For this review, use the dimensioned drawing (mm, ordinates from the lowest corner) and the shaded views. Round coordinates to 2 decimals unless told otherwise and drop trailing zeros. Loops run counter-clockwise (first coordinate to the right, second up) from the corner with the lowest first, then second, coordinate; pieces in that order, holes last. Notation, with made-up numbers: M 89,44 L 108,44 A29 cw 108,65 Z; hole C 72,31.25 d11. An arc over 180 degrees is marked long. Answer as a JSON object with one key per item and string values. Group by question number.
Item 1: Consider section B-B (x = 45). Give the boundary of the cut face in (y, z), and give its area (3 significant figures).
Item 2: Insertion check: P1, Ø1.2, axis at x = 60, y = 34, coming from the +Z side; P2, Ø2.5, axis at x = 115, y = 2, coming from the +Z side; P3, Ø0.8, axis at x = 68.5, z = 2.5, coming from the +Y side. Each pin has a flat end and moves straight along its axis. Give the tip position at first contact, or say it passes through.
Item 3: To check wall thickness, follow line 1 (X direction, y = 34, z = 0.8); line 2 (Y direction, x = 60, z = 1.6); line 3 (Z direction, x = 42, y = 4). State the ranges of each line that lie inside material, in increasing order.
Item 4: Consider section A-A (y = 8). Give the boundary of the cut face in (x, z).
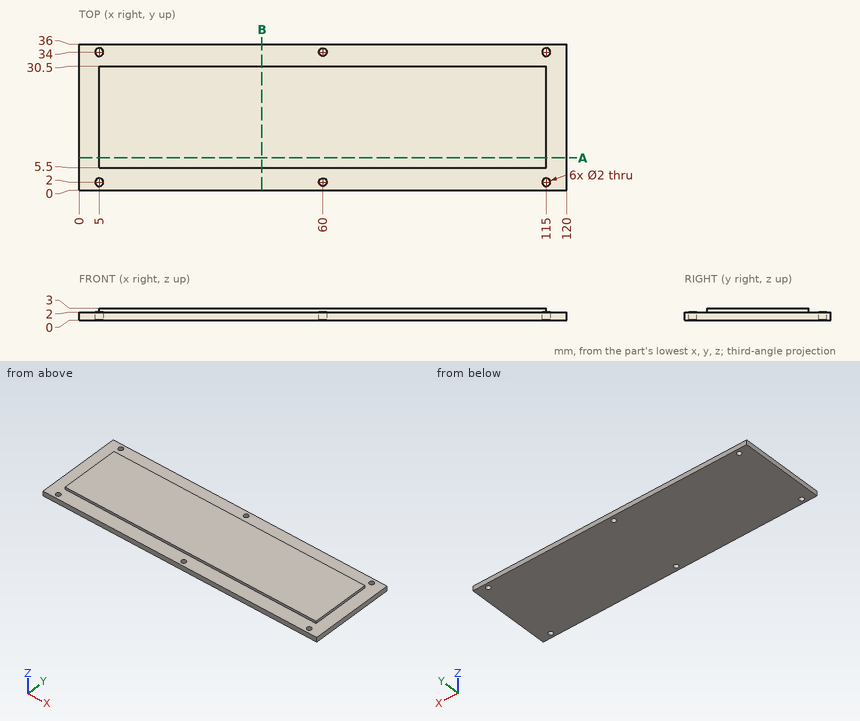
Geometry results:
{
 "1": {"outline": "M 0,0 L 36,0 L 36,2 L 30.5,2 L 30.5,3 L 5.5,3 L 5.5,2 L 0,2 Z", "area": "97.0 mm^2"},
 "2": {"P1": "passes through", "P2": "stops at z = 2", "P3": "stops at y = 30.5"},
 "3": {"line 1": "x = 0 to 4, 6 to 59, 61 to 114, 116 to 120", "line 2": "y = 0 to 1, 3 to 33, 35 to 36", "line 3": "z = 0 to 2"},
 "4": {"outline": "M 0,0 L 120,0 L 120,2 L 115,2 L 115,3 L 5,3 L 5,2 L 0,2 Z"}
}
